Geometry check sheet. Reference: the model listing, model coordinates, mm. Give positions to 0.01 mm unless a question says otherwise; leave off trailing zeros. Order: outer loops, then holes, each group sorted by start corner. A loop starts at its lowest first (then second) coordinate and runs counter-clockwise, first axis right, second up.
```python
from build123d import *

# Parameters (mm, degrees)
ESBO_O1_R                = 4.05
ESBO_O1_R_2              = 2.574080602
RESSALTO_EXTRUS_O1_DEPTH = 1.5
FILETE1_R                = 1.5


with BuildPart() as part:
    # Esboço1 → Ressalto-extrusão1 (new body)
    with BuildSketch(Plane.XY):
        with BuildLine():
            Line((-18.018564211, 0), (-18.018564211, -8))
            ThreePointArc((-18.018564211, -8), (-19.612515049, -14.728881473), (-24.055610328, -20.027695444))
            Line((-24.055610328, -20.027695444), (-110.751402368, -20.027695444))
            Line((-110.751402368, -20.027695444), (-90.563626469, -45.733186479))
            Line((-90.563626469, -45.733186479), (-19.714622268, -45.733186479))
            ThreePointArc((-19.714622268, -45.733186479), (6.966769767, -34.681392035), (18.018564211, -8))
            Line((18.018564211, -8), (18.018564211, 0))
            ThreePointArc((18.018564211, 0), (0, 18.018564211), (-18.018564211, 0))
        make_face()
        Circle(ESBO_O1_R, mode=Mode.SUBTRACT)
        with Locations((-58.195334888, -25.027695444)):
            Circle(ESBO_O1_R_2, mode=Mode.SUBTRACT)
        with Locations((-58.195334888, -40.733186479)):
            Circle(ESBO_O1_R_2, mode=Mode.SUBTRACT)
        with Locations((-92.935045512, -31.639829044)):
            Circle(ESBO_O1_R, mode=Mode.SUBTRACT)
    extrude(amount=RESSALTO_EXTRUS_O1_DEPTH)

    # Filete1
    filete1_edges = [part.edges().sort_by_distance(p)[0] for p in [
        (-110.751402368, -20.027695444, 0.75),
    ]]
    fillet(filete1_edges, radius=FILETE1_R)


solid = part.part
```
Q1. Thickness scan on L1, parallel to X at y = -6.5, z = 0.35; L2, parallel to Y at x = 0, z = 0.9; L3, parallel to X at y = 3, z = 0.35. Record the ranges inside material, lowest first.
Q2. Cross-section at B-B, the plane x = 2.5. Record the boundary of the cut face in (y, z), and give its area (3 significant figures).
Q3. Gauge pin test, flat end, axial feed: P1, Ø0.8, axis at y = -5.5, z = 1, coming from the -X side. Record the tip position at first contact, or that the pin passes through.
Q4. Cross-section at C-C, the plane x = -72. Record the boundary of the cut face in (y, z).
Q5. Release check for a two-part mould opening along X. For faces 1 (the face through (-32.3, -20.5, 0)), 2 (the face through (-0.878, -3.954, 0.74)), 3 (the face through (0.396, 18.014, 0.74)) record: pulls with the +X half, pulls with the -X half, needs draft (parallel to the pull), parting line crosses it, or undercut.
Q6. Cross-section at D-D, the plane y = -14.5. Record the boundary of the cut face in (x, z).
Q7. Cross-section at A-A, the plane z = 1.1. Record the boundary of the cut face in (x, y).
Answers follow:
1. L1: x = -18.02 to 18.02
1. L2: y = -40.17 to -4.05, 4.05 to 18.02
1. L3: x = -17.77 to -2.72, 2.72 to 17.77
2. outline: (-38.5, 0) - (-3.19, 0) - (-3.19, 1.5) - (-38.5, 1.5) - close; (3.19, 0) - (17.84, 0) - (17.84, 1.5) - (3.19, 1.5) - close
2. area: 75.0 mm2
3. P1: stops at x = -18.02
4. outline: (-45.73, 0) - (-20.03, 0) - (-20.03, 1.5) - (-45.73, 1.5) - close
5. face 1: needs draft
5. face 2: undercut
5. face 3: parting line crosses it
6. outline: (-19.5, 0) - (17.45, 0) - (17.45, 1.5) - (-19.5, 1.5) - close
7. outline: (-108.85, -22.45) - (-90.56, -45.73) - (-19.71, -45.73) arc R37.73 ccw to (18.02, -8) - (18.02, 0) arc R18.02 ccw to (-18.02, 0) - (-18.02, -8) arc R15 cw to (-24.06, -20.03) - (-107.67, -20.03) arc R1.5 ccw to start; hole circle Ø8.1 at (-92.94, -31.64); hole circle Ø5.15 at (-58.2, -40.73); hole circle Ø5.15 at (-58.2, -25.03); hole circle Ø8.1 at (0, 0)
